```python
from build123d import *

# Parameters (mm, degrees)
SKETCH1_W            = 7.1
SKETCH1_H            = 6.5
BOSS_EXTRUDE1_DEPTH  = 2.85
CHAMFER1_SIZE        = 1.5
FILLET1_R            = 1
SKETCH2_W            = 0.9
SKETCH2_H            = 2.7
CUT_EXTRUDE1_DEPTH   = 0.3
SKETCH3_W            = 0.5
SKETCH3_H            = 3.2
CUT_EXTRUDE2_DEPTH   = 0.3
FILLET2_R            = 0.25
FILLET2_OF_MIRROR1_R = 0.25


with BuildPart() as part:
    # Sketch1 → Boss-Extrude1 (new body)
    with BuildSketch(Plane(origin=(0, 0, 0), x_dir=(1, 0, 0), z_dir=(0, 1, 0))):
        Rectangle(SKETCH1_W, SKETCH1_H)
    extrude(amount=BOSS_EXTRUDE1_DEPTH)

    # Chamfer1
    chamfer1_edges = [part.edges().sort_by_distance(p)[0] for p in [
        (3.55, 1.425, 3.25),
        (-3.55, 1.425, -3.25),
    ]]
    chamfer(chamfer1_edges, length=CHAMFER1_SIZE)

    # Fillet1
    fillet1_edges = [part.edges().sort_by_distance(p)[0] for p in [
        (-3.55, 1.425, 3.25),
        (3.55, 1.425, -3.25),
    ]]
    fillet(fillet1_edges, radius=FILLET1_R)

    # Sketch2 → Cut-Extrude1 (cut)
    with BuildSketch(Plane(origin=(0, 2.85, 0), x_dir=(1, 0, 0), z_dir=(0, 1, 0))):
        with Locations((3.1, 0)):
            Rectangle(SKETCH2_W, SKETCH2_H)
    cut_extrude1 = extrude(amount=-CUT_EXTRUDE1_DEPTH, mode=Mode.SUBTRACT)

    # Sketch3 → Cut-Extrude2 (cut)
    with BuildSketch(Plane(origin=(0, 2.85, 0), x_dir=(1, 0, 0), z_dir=(0, 1, 0))):
        with Locations((2.4, 0)):
            Rectangle(SKETCH3_W, SKETCH3_H)
    cut_extrude2 = extrude(amount=-CUT_EXTRUDE2_DEPTH, mode=Mode.SUBTRACT)

    # Fillet2
    fillet2_edges = [part.edges().sort_by_distance(p)[0] for p in [
        (2.65, 2.7, 1.6),
        (2.15, 2.7, 1.6),
        (2.65, 2.7, -1.6),
        (2.15, 2.7, -1.6),
    ]]
    fillet(fillet2_edges, radius=FILLET2_R - 0.0001)  # a hair under: the kernel refuses the full size

    # Mirror1: Cut-Extrude1, Cut-Extrude2 across plane
    add(cut_extrude1.mirror(Plane(origin=(0, 0, 0), x_dir=(0, 0, 1), z_dir=(1, 0, 0))), mode=Mode.SUBTRACT)
    add(cut_extrude2.mirror(Plane(origin=(0, 0, 0), x_dir=(0, 0, 1), z_dir=(1, 0, 0))), mode=Mode.SUBTRACT)

    # Fillet2 of Mirror1
    fillet2_of_mirror1_edges = [part.edges().sort_by_distance(p)[0] for p in [
        (-2.65, 2.7, 1.6),
        (-2.15, 2.7, 1.6),
        (-2.65, 2.7, -1.6),
        (-2.15, 2.7, -1.6),
    ]]
    fillet(fillet2_of_mirror1_edges, radius=FILLET2_OF_MIRROR1_R - 0.0001)  # a hair under: the kernel refuses the full size


solid = part.part
```
Input: part model. Units: mm. Frame: model coordinates. Round coordinates to 2 decimals unless told otherwise and drop trailing zeros. Write each loop counter-clockwise with the first axis right and the second up, starting at its lowest first coordinate (ties: lowest second). Pieces come first, ordered by that corner, then holes. Notation, with made-up numbers: (-40, 31.5) - (-5, 31.5) arc R14 ccw to (-5, 50.5) - close; hole circle Ø1 at (11.5, 14.25). An arc over 180 degrees is marked (long way). Write item = value, one per line.
(1) Contact query for a flat-ended pin moving along its axis: pin 1 Ø0.7 at (x, z) = (3, 0) entering from +Y. Output: stop coordinate, or through.
Geometry check:
pin_1 = 2.55
(2) Material intervals for probe 1 along Y at (x, z) = (2.5, -1); probe 2 along X at (y, z) = (2.65, 0); probe 3 along X at (y, z) = (1.65, -2.5), sorted ascending.
Geometry check:
probe_1 = 0 to 2.55
probe_2 = -2.15 to 2.15
probe_3 = -2.8 to 3.52
(3) Section query B-B on y = 2.15. Output: boundary loops of the cut face in (x, z), then the cut area to 3 significant figures.
Geometry check:
outline = (-3.55, -1.75) - (-2.05, -3.25) - (2.55, -3.25) arc R1 ccw to (3.55, -2.25) - (3.55, 1.75) - (2.05, 3.25) - (-2.55, 3.25) arc R1 ccw to (-3.55, 2.25) - close
area = 43.5 mm^2
(4) Section query C-C on z = -2.5. Output: boundary loops of the cut face in (x, y), then the cut area to 3 significant figures.
Geometry check:
outline = (-2.8, 0) - (3.52, 0) - (3.52, 2.85) - (-2.8, 2.85) - close
area = 18.0 mm^2
(5) Pull-direction query (Z, two-part tool) for faces 1 (the flat face through (-3.55, 1, 0)), 2 (the flat face through (0, 1, -3.25)), 3 (the flat face through (3, 2.55, 0)); classes: +Z half, -Z half, draft (parallel to the pull), parting line (faces both ways), or undercut.
Geometry check:
face_1 = draft
face_2 = -Z half
face_3 = undercut
(6) Section query A-A on z = 0.75. Output: boundary loops of the cut face in (x, y), then the cut area to 3 significant figures.
Geometry check:
outline = (-3.55, 0) - (3.55, 0) - (3.55, 2.55) - (2.15, 2.55) - (2.15, 2.85) - (-2.15, 2.85) - (-2.15, 2.55) - (-3.55, 2.55) - close
area = 19.4 mm^2
